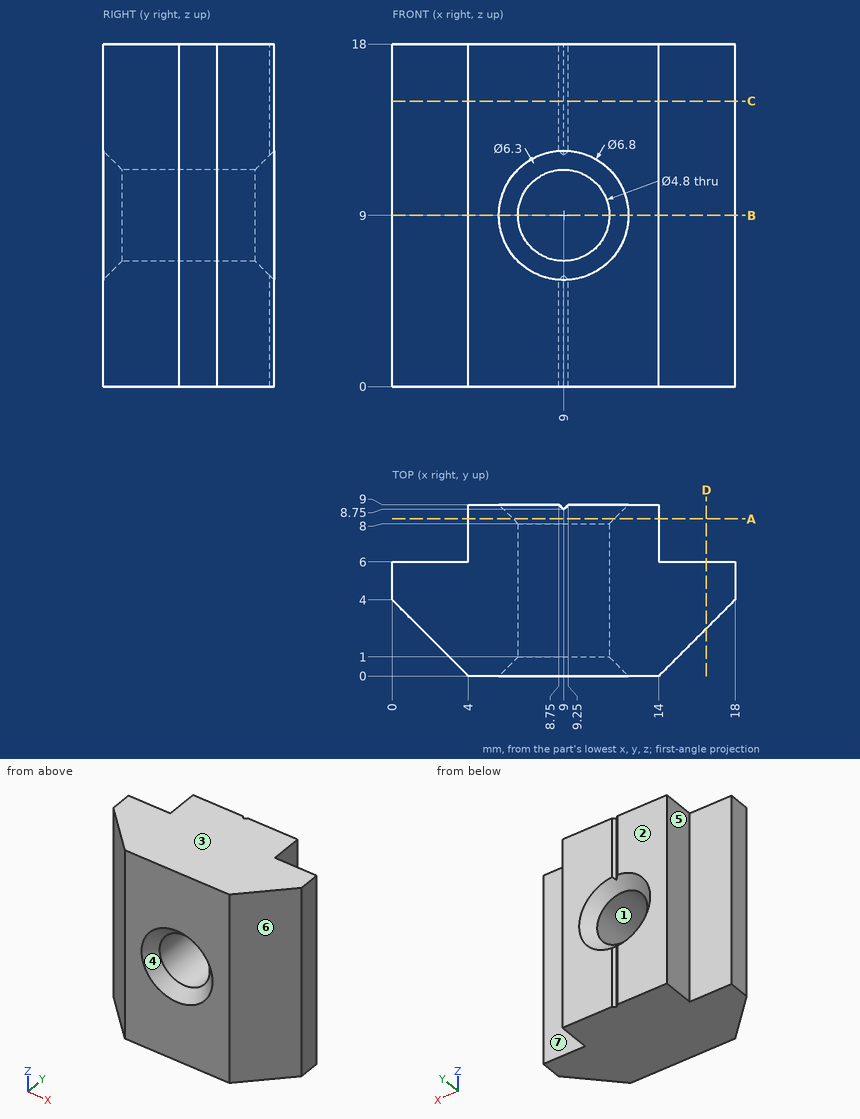
Here's the drawing with two shaded views (mm, measured from the low corner). I have some questions. A direction names the side the tool comes from. Round coordinates to 2 decimals unless told otherwise and drop trailing zeros. Loops run counter-clockwise (first coordinate to the right, second up) from the corner with the lowest first, then second, coordinate; pieces in that order, holes last.
1. Suppose I cut it at B-B, the plane z = 9. Please give me the cut outline in (x, y), and give its area (3 significant figures).
Answers:
outline: (0, 4) - (4, 0) - (5.6, 0) - (6.6, 1) - (6.6, 8) - (5.6, 9) - (4, 9) - (4, 6) - (0, 6) - close; (11.4, 1) - (12.4, 0) - (14, 0) - (18, 4) - (18, 6) - (14, 6) - (14, 9) - (12.4, 9) - (11.4, 8) - close
area: 76.8 mm2
2. For the marked faces 5, 6 and 7, which set-ups out of +Z, -Z, +X, -X, +Y, -Y let a thin tool reach every point of the face, with its end or its side?
Answers:
face 5: +Z, -Z, -X, +Y
face 6: +Z, -Z, +X, -Y
face 7: +Z, -Z, +X, +Y
3. Will these pins go through, and if not, where does the flat tip stop? pin 1 (0.9 mm diameter, centred on y = 7.5, z = 11, fed in from +X); pin 2 (2 mm diameter, centred on x = 15.5, z = 8, fed in from +Y); pin 3 (3 mm diameter, centred on y = 1.5, z = 6, fed in from +X); pin 4 (5 mm diameter, centred on y = 6.5, z = 6, fed in from -X).
Answers:
pin 1: stops at x = 14
pin 2: stops at y = 6
pin 3: stops at x = 17
pin 4: stops at x = 0
4. If I drill on probe 1 along Z at (x, y) = (9, 4.25); probe 2 along X at (y, z) = (6.25, 9), over which ranges is the centre line in solid material (lowest first)?
Answers:
probe 1: z = 0 to 6.6, 11.4 to 18
probe 2: x = 4 to 6.6, 11.4 to 14
5. Suppose I cut it at C-C, the plane z = 15. Please give me the cut outline in (x, y).
Answers:
outline: (0, 4) - (4, 0) - (14, 0) - (18, 4) - (18, 6) - (14, 6) - (14, 9) - (9.25, 9) - (9, 8.75) - (8.75, 9) - (4, 9) - (4, 6) - (0, 6) - close
6. Thinking about a two-plate mould opening in Z: for the marked faces 1, 2, 3 and 4, which applies, released by +Z, released by -Z, zero draft, split by the parting line, or undercut?
Answers:
face 1: undercut
face 2: zero draft
face 3: released by +Z
face 4: undercut
7. Suppose I cut it at D-D, the plane x = 16.5. Please give me the cut outline in (y, z), and give its area (3 significant figures).
Answers:
outline: (2.5, 0) - (6, 0) - (6, 18) - (2.5, 18) - close
area: 63.0 mm2
8. Suppose I cut it at A-A, the plane y = 8.25. Please give me the cut outline in (x, z).
Answers:
outline: (4, 0) - (14, 0) - (14, 18) - (4, 18) - close; hole circle Ø5.3 at (9, 9)
